Here's how the part is built. I have some questions about the finished solid (model axes, mm). Face numbers are marked on the shaded views. A direction names the side the tool comes from. Round coordinates to 2 decimals unless told otherwise and drop trailing zeros. Loops run counter-clockwise (first coordinate to the right, second up) from the corner with the lowest first, then second, coordinate; pieces in that order, holes last. Notation, with made-up numbers: M -33,5.25 L 11,5.25 A5 ccw 11,12.25 Z; hole C 63,14 d3. An arc over 180 degrees is marked long. Answer as a JSON object with one key per item and string values.
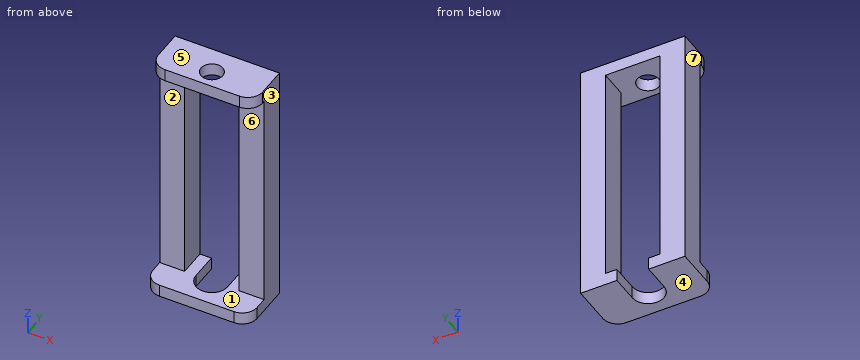
Autodesk Inventor part; units mm, degrees
ref_plane "YZ Plane" through (0, 0, 0) normal (1, 0, 0) x (0, 1, 0)
ref_plane "XZ Plane" through (0, 0, 0) normal (0, 1, 0) x (-1, 0, 0)
ref_plane "XY Plane" through (0, 0, 0) normal (0, 0, 1) x (1, 0, 0)
sketch "Sketch1" plane through (0, 0, 0) normal (0, 0, 1) x (1, 0, 0)
  arc A0 (-3.2, 0) -> (3.2, 0) centre (0, 0) ccw
  arc A1 (-5.5, 0) -> (5.5, 0) centre (0, 0) ccw
  line L0 (-3.2, 0) -> (-5.5, 0)
  line L1 (-5.5, 0) -> (-5.5, 5.5)
  line L2 (-5.5, 5.5) -> (-3.2, 5.5)
  line L3 (-3.2, 5.5) -> (-3.2, 0)
  line L4 (3.2, 0) -> (5.5, 0)
  line L5 (5.5, 0) -> (5.5, 5.5)
  line L6 (5.5, 5.5) -> (3.2, 5.5)
  line L7 (3.2, 5.5) -> (3.2, 0)
  line L8 (-5.5, 0) -> (-5.5, 5.5)
  line L9 (-5.5, 5.5) -> (-10.5, 5.5)
  line L10 (-10.5, 5.5) -> (-10.5, 0)
  line L11 (-10.5, 0) -> (-5.5, 0)
  line L12 (5.5, 0) -> (5.5, 5.5)
  line L13 (5.5, 5.5) -> (10.5, 5.5)
  line L14 (10.5, 5.5) -> (10.5, 0)
  line L15 (10.5, 0) -> (5.5, 0)
  line L16 (10.5, 0) -> (10.5, -5.5)
  line L17 (10.5, -5.5) -> (-10.5, -5.5)
  line L18 (-10.5, -5.5) -> (-10.5, 0)
  dimension "d0" = 6.4
  dimension "d1" = 11
  dimension "d2" = 5
  dimension "d3" = 5
extrude "Extr-legs" add sketch "Sketch1" along normal blind 45 contours L11 L10 L9 L1 | L5 L13 L14 L15
extrude "Extr-base" add sketch "Sketch1" against normal blind 2.5 contours A0 L4 A1 L0 | L0 L1 L2 L3 | L7 L6 L5 L4 | L11 L10 L9 L1 | L5 L13 L14 L15
sketch "Sketch2" plane through (0, 0, 45) normal (0, 0, 1) x (1, 0, 0)
  circle A0 centre (0, 0) radius 2.2
  circle A1 centre (0, 0) radius 3.5
  line L0 (5.5, 0) -> (10.5, 0)
  line L1 (-10.5, 0) -> (-5.5, 0)
  line L2 (-10.5, 0) -> (-10.5, 5.5)
  line L3 (-10.5, 5.5) -> (10.5, 5.5)
  line L4 (10.5, 5.5) -> (10.5, 0)
  line L5 (10.5, 0) -> (2.2, 0)
  line L6 (-2.2, 0) -> (-10.5, 0)
  line L7 (-10.5, 0) -> (-10.5, -3.5)
  line L8 (-10.5, -3.5) -> (10.5, -3.5)
  line L9 (10.5, -3.5) -> (10.5, 0)
  dimension "d8" = 4.4
  dimension "d9" = 7
extrude "Extr-top" add sketch "Sketch2" along normal blind 2.5 contours L5 A1 L6 A0 | A0 L6 A1 L5 | L5 L0 L9 L8 A1 | A1 L6 L1 L2 L3 L4 L0 L5 | A1 L8 L7 L1 L6
extrude "Extrusion4" add sketch "Sketch1" against normal up to surface (2.5 mm away) contours A1 L17 L18 L11 | L15 L16 L17 A1
fillet "Fillet1" radius 3 4 edges at (10.5, -3.5, 46.25) (10.5, -5.5, -1.25) (-10.5, -3.5, 46.25) (-10.5, -5.5, -1.25)
properties part number "cage2table-mount-M4(top)-M6(bottom)"
Item 1: I want a section at A-A, the plane x = -5. Please give me the cut outline in (y, z), then the cut area to 3 significant figures.
Resolved:
{"outline": "M -5.5,-2.5 L 5.5,-2.5 L 5.5,0 L -5.5,0 Z; M -3.5,45 L 5.5,45 L 5.5,47.5 L -3.5,47.5 Z", "area": "50.0 mm²"}
Item 2: If we mould it in two halves opening along Z, with no side actions, what happens to the marked faces 4, 5, 6 and 7? For each: pulls with the +Z half, pulls with the -Z half, needs draft (parallel to the pull), parting line crosses it, or undercut.
Resolved:
{"face 4": "pulls with the -Z half", "face 5": "pulls with the +Z half", "face 6": "undercut", "face 7": "needs draft"}
Item 3: I'm going to push flat-ended pins straight in: pin 1 Ø5 at (x, y) = (0, 0) entering from -Z; pin 2 Ø6 at (x, z) = (-3.5, 39) entering from -Y; pin 3 Ø3 at (y, z) = (-2, 33.5) entering from +X; pin 4 Ø1.2 at (x, z) = (1.5, 45.5) entering from -Y. Where does each tip first touch, or does it pass through?
Resolved:
{"pin 1": "z = 45", "pin 2": "y = 0", "pin 3": "through", "pin 4": "y = -3.5"}
Item 4: Please list where these lines run through material, in increasing order: probe 1 along Z at (x, y) = (8, -0.5); probe 2 along X at (y, z) = (5, 5); probe 3 along X at (y, z) = (0, 46.6). Write a range as from..to.
Resolved:
{"probe 1": "-2.5..0, 45..47.5", "probe 2": "-10.5..-5.5, 5.5..10.5", "probe 3": "-10.5..-2.2, 2.2..10.5"}
Item 5: I want a section at B-B, the plane x = 0. Please give me the cut outline in (y, z), then the cut area to 4 significant figures.
Resolved:
{"outline": "M -5.5,-2.5 L -3.2,-2.5 L -3.2,0 L -5.5,0 Z; M -3.5,45 L -2.2,45 L -2.2,47.5 L -3.5,47.5 Z; M 2.2,45 L 5.5,45 L 5.5,47.5 L 2.2,47.5 Z", "area": "17.25 mm²"}
Item 6: I want a section at C-C, the plane z = 35. Please give me the cut outline in (x, y), then the cut area to 3 significant figures.
Resolved:
{"outline": "M -10.5,0 L -5.5,0 L -5.5,5.5 L -10.5,5.5 Z; M 5.5,0 L 10.5,0 L 10.5,5.5 L 5.5,5.5 Z", "area": "55.0 mm²"}
Item 7: On a 3-axis mill with a long thin cutter (end or side, diameter ignored), from which of +Z, -Z, +X, -X, +Y, -Y can I reach the whole of each face in a straight line? I mean the marked faces 1, 2 and 3. Say none if no direction works.
Resolved:
{"face 1": "-Y", "face 2": "+X, -X, -Y", "face 3": "+Z, -Z, +X, +Y, -Y"}
Item 8: I want a section at D-D, the plane y = 2.75. Please give me the cut outline in (x, z).
Resolved:
{"outline": "M -10.5,-2.5 L -3.2,-2.5 L -3.2,0 L -5.5,0 L -5.5,45 L 5.5,45 L 5.5,0 L 3.2,0 L 3.2,-2.5 L 10.5,-2.5 L 10.5,47.5 L -10.5,47.5 Z"}
